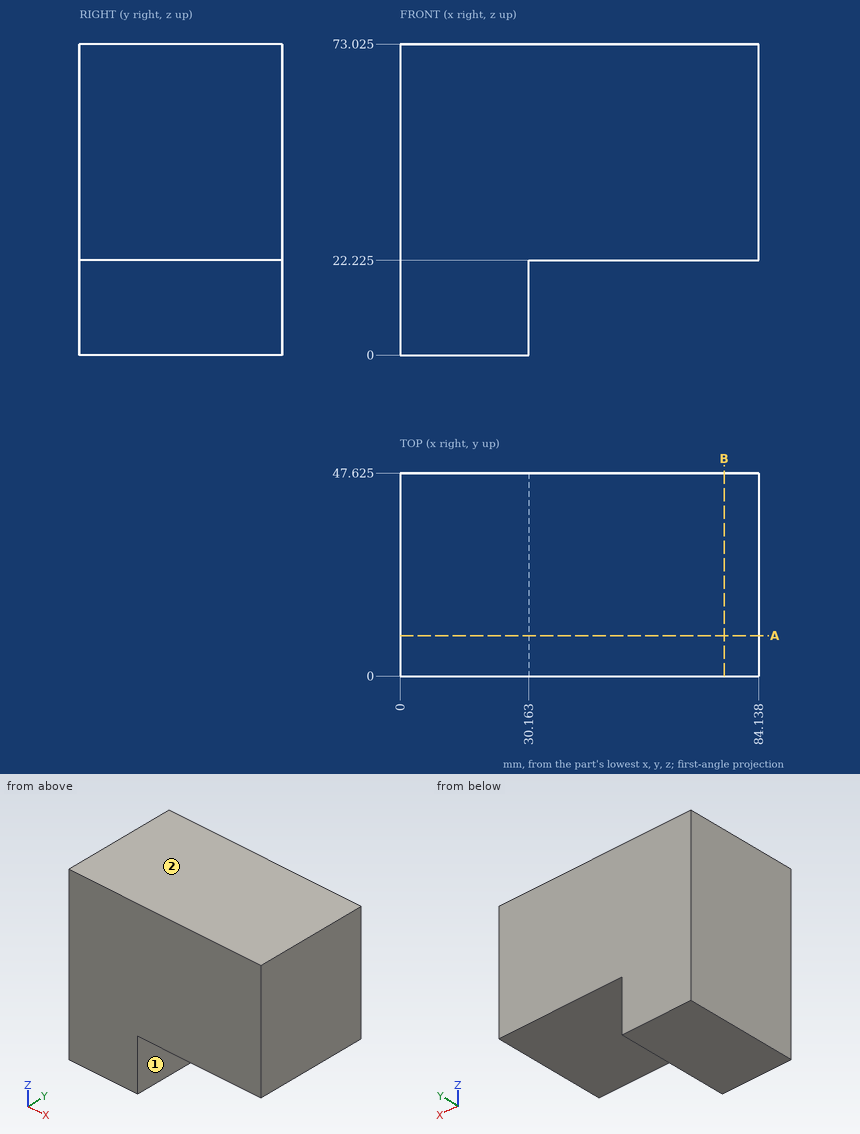
Source: three-view drawing plus pictorial views. Frame: mm from the lowest corner of the part. A direction names the side the tool comes from. Coordinates: 2 decimals unless noted, no trailing zeros. Loops run counter-clockwise (first coordinate to the right, second up) from the corner with the lowest first, then second, coordinate; pieces in that order, holes last. Notation, with made-up numbers: (-22.75, 10) -> (-8.75, 10) arc R16 cw to (-8.75, 29) -> close; hole circle Ø4 at (-5, 55.25). An arc over 180 degrees is marked (long way). Write each question's results on one line, items separated by ' | '. Start each with the question number.
Q1. Pin query (flat end, axial travel): pin 1 (2 mm diameter, centred on x = 75, y = 22, fed in from -Z) (1 decimal); pin 2 (12 mm diameter, centred on x = 41, z = 19.5, fed in from -Y); pin 3 (24.5 mm diameter, centred on y = 31.5, z = 7.5, fed in from +X). Return the tip coordinate at first contact, or that it passes through.
Q2. Section B-B, the plane x = 76. Return the cut outline in (y, z) (1 decimal).
Q3. Section A-A, the plane y = 9.5. Return the cut outline in (x, z) (1 decimal), plus the area to 3 significant figures.
Q4. Ray query, line 1 (Z direction, x = 69.5, y = 23) (1 decimal); line 2 (X direction, y = 43.5, z = 10). Return the intervals inside material, ascending. Write a range as from..to.
Q5. Reachability of the marked faces 1 and 2 from +Z, -Z, +X, -X, +Y, -Y: full face, straight path, thin tool, end or side. Return the list, or none.
Found:
1) pin 1: z = 22.2 | pin 2: y = 0 | pin 3: x = 30.16
2) outline: (0, 22.2) -> (47.6, 22.2) -> (47.6, 73) -> (0, 73) -> close
3) outline: (0, 0) -> (30.2, 0) -> (30.2, 22.2) -> (84.1, 22.2) -> (84.1, 73) -> (0, 73) -> close | area: 4,940 mm2
4) line 1: 22.2..73 | line 2: 0..30.16
5) face 1: -Z, +X, +Y, -Y | face 2: +Z, +X, -X, +Y, -Y
